from build123d import *

# Parameters (mm, degrees)
F1_DEPTH = 12.7


with BuildPart() as f1:
    # F0 (on Top) → F1 (new body)
    with BuildSketch(Plane.XY):
        Polygon((8.306665788, 14.6107980981), (-20.214330405, 14.6107980981), (-20.214330405, -14.5559702069), (18.9034491777, -14.5559702069), (18.9034491777, 14.6107980981), (13.2803532164, 14.6107980981), (16.125800088, 12.2895119712), (9.568403475, -5.3119254299), (3.5286939237, 3.1436665449), align=None)
        Polygon((-20.214330405, -14.5559702069), (-20.214330405, 14.6107980981), (-23.4641304458, 12.2895119712), (-23.4641304458, -17.2187797725), align=None)
        Polygon((9.568403475, 17.6389683038), (8.306665788, 14.6107980981), (13.2803532164, 14.6107980981), align=None)
        Polygon((13.2803532164, 14.6107980981), (8.306665788, 14.6107980981), (3.5286939237, 3.1436665449), (9.568403475, -5.3119254299), (16.125800088, 12.2895119712), align=None)
        Polygon((18.9034491777, -14.5559702069), (-20.214330405, -14.5559702069), (-23.4641304458, -17.2187797725), (16.125800088, -17.2187797725), align=None)
    extrude(amount=F1_DEPTH)


solid = f1.part
Can you work these out from the model? Positions are in its coordinate system, mm. A direction names the side the tool comes from. Give positions to 0.01 mm unless a question says otherwise; leave off trailing zeros. Write each loop counter-clockwise with the first axis right and the second up, starting at its lowest first coordinate (ties: lowest second). Pieces come first, ordered by that corner, then holes. Notation, with made-up numbers: (-36, 84.25) -> (-2, 84.25) arc R6 cw to (-2, 90.25) -> close; hole circle Ø3 at (82.5, 76.5). An arc over 180 degrees is marked (long way). Answer as a JSON object with one key per item and string values. Group by question number.
Item 1: For faces 1 (the face through (-6, 14.611, 6)), 2 (the face through (17.5, -15.9, 6.3)), 3 (the face through (16, 14.611, 6)), which set-ups out of +Z, -Z, +X, -X, +Y, -Y let a thin tool reach every point of the face, with its end or its side?
Item 2: I'm going to push a flat-ended pin straight in: P1, Ø4, axis at x = -10, z = 4.5, coming from the +Y side. Where does the tip first touch, or does it pass through?
Item 3: Suppose I cut it at B-B (x = -5.5). Please give me the cut outline in (y, z), plus the area to 3 significant figures.
Item 4: Suppose I cut it at A-A (z = 8). Please give me the cut outline in (x, y), plus the area to 3 significant figures.
Item 5: Please list where these lines run through material, in increasing order: line 1 (Y direction, x = 6, z = 8.75); line 2 (X direction, y = 14.5, z = 2.75). Write a range as [from, to].
Findings:
{
 "1": {"face 1": "+Z, -Z, -X, +Y", "face 2": "+Z, -Z, +X, -Y", "face 3": "+Z, -Z, +X, +Y"},
 "2": {"P1": "stops at y = 14.61"},
 "3": {"outline": "(-17.22, 0) -> (14.61, 0) -> (14.61, 12.7) -> (-17.22, 12.7) -> close", "area": "404 mm²"},
 "4": {"outline": "(-23.46, -17.22) -> (16.13, -17.22) -> (18.9, -14.56) -> (18.9, 14.61) -> (13.28, 14.61) -> (9.57, 17.64) -> (8.31, 14.61) -> (-20.21, 14.61) -> (-23.46, 12.29) -> close", "area": "1,350 mm²"},
 "5": {"line 1": "y = [-17.22, 14.61]", "line 2": "x = [-20.37, 18.9]"}
}
